Input: dimensioned drawing with shaded views. Units: mm. Origin: part minimum x, y, z. A direction names the side the tool comes from. Coordinates: 2 decimals unless noted, no trailing zeros. Loops run counter-clockwise (first coordinate to the right, second up) from the corner with the lowest first, then second, coordinate; pieces in that order, holes last.
Item 1: Section C-C on x = 4. Return loops of the section in (y, z).
Item 2: Section A-A on x = 56. Return loops of the section in (y, z).
Item 3: Contact query for flat-ended pins moving along their axis: P1, Ø1, axis at y = 11, z = 0.5, coming from the -X side; P2, Ø2.5, axis at x = 56, z = 2.5, coming from the -Y side. Output: stop coordinate, or through.
Item 4: Pull-direction query (Y, two-part tool) for the marked faces 4, 5 and 6; classes: released by +Y, released by -Y, zero draft, split by the parting line, or undercut.
Item 5: Section D-D on z = 1.3. Return loops of the section in (x, y).
Item 6: Reachability of the marked faces 1, 2 and 3 from +Z, -Z, +X, -X, +Y, -Y: full face, straight path, thin tool, end or side. Return the list, or none.
Item 7: Section B-B on y = 29. Return loops of the section in (x, z).
Item 8: Ray query, line 1 along Y through (x, z) = (4, 3.2); line 2 along Y through (x, z) = (31, 1.45); line 3 along X through (y, z) = (27.5, 4.25). Return the intervals inside material, ascending.
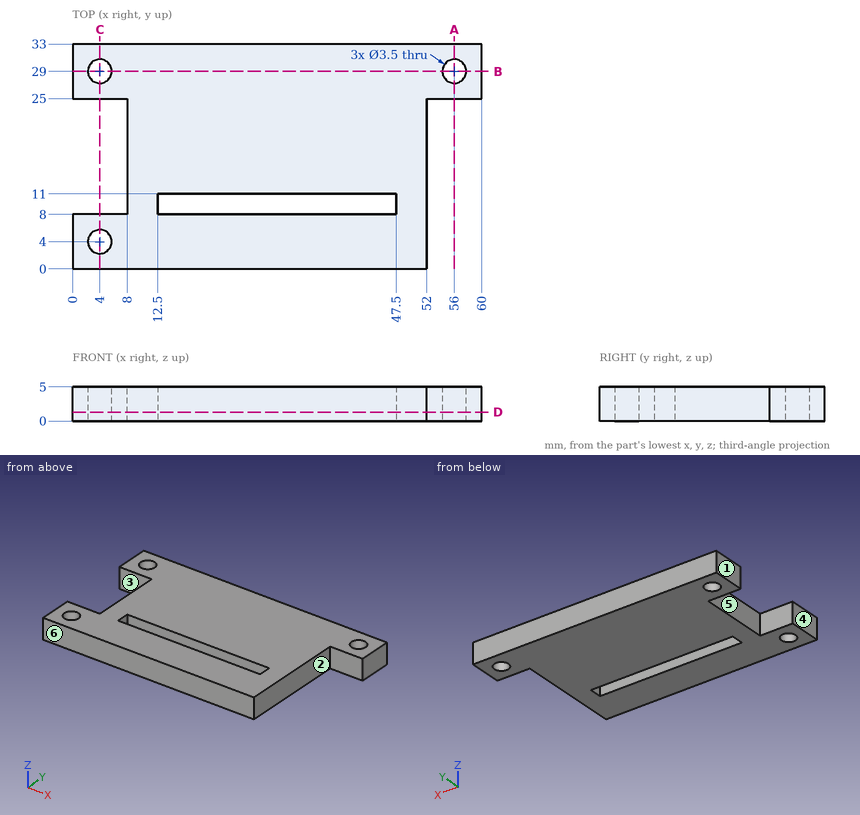
Results found:
1. outline: (0, 0) - (2.25, 0) - (2.25, 5) - (0, 5) - close; (5.75, 0) - (8, 0) - (8, 5) - (5.75, 5) - close; (25, 0) - (27.25, 0) - (27.25, 5) - (25, 5) - close; (30.75, 0) - (33, 0) - (33, 5) - (30.75, 5) - close
2. outline: (25, 0) - (27.25, 0) - (27.25, 5) - (25, 5) - close; (30.75, 0) - (33, 0) - (33, 5) - (30.75, 5) - close
3. P1: stops at x = 8
3. P2: stops at y = 25
4. face 4: zero draft
4. face 5: undercut
4. face 6: released by -Y
5. outline: (0, 0) - (52, 0) - (52, 25) - (60, 25) - (60, 33) - (0, 33) - (0, 25) - (8, 25) - (8, 8) - (0, 8) - close; hole circle Ø3.5 at (4, 4); hole circle Ø3.5 at (4, 29); hole (12.5, 8) - (47.5, 8) - (47.5, 11) - (12.5, 11) - close; hole circle Ø3.5 at (56, 29)
6. face 1: +Z, -Z, -X, +Y, -Y
6. face 2: +Z, -Z, +X, -Y
6. face 3: +Z, -Z, -X
7. outline: (0, 0) - (2.25, 0) - (2.25, 5) - (0, 5) - close; (5.75, 0) - (54.25, 0) - (54.25, 5) - (5.75, 5) - close; (57.75, 0) - (60, 0) - (60, 5) - (57.75, 5) - close
8. line 1: y = 0 to 2.25, 5.75 to 8, 25 to 27.25, 30.75 to 33
8. line 2: y = 0 to 8, 11 to 33
8. line 3: x = 0 to 3.1, 4.9 to 55.1, 56.9 to 60
